from build123d import *

# Parameters (mm, degrees)
ESQUISSE1_R      = 2.5
ESQUISSE1_R_2    = 9
ESQUISSE1_R_3    = 2
EXTRUSION1_DEPTH = 3
CONG_1_R         = 15
EXTRUSION2_REACH = 5
ESQUISSE2_W      = 300
ESQUISSE2_H      = 3
ESQUISSE2_W_2    = 3
ESQUISSE2_H_2    = 91
ESQUISSE2_H_3    = 79
EXTRUSION3_REACH = 5
ESQUISSE3_R      = 2.5


with BuildPart() as part:
    # Esquisse1 → Extrusion1 (new body)
    with BuildSketch(Plane(origin=(0, 0, 0), x_dir=(1, 0, 0), z_dir=(0, 1, 0))):
        Polygon((0, 0), (24, 0), (24, 117), (165, 117), (306, 117), (306, 0), (330, 0), (330, 210), (0, 210), align=None)
        with Locations((10, 200)):
            Circle(ESQUISSE1_R, mode=Mode.SUBTRACT)
        with Locations((320, 200)):
            Circle(ESQUISSE1_R, mode=Mode.SUBTRACT)
        with Locations((10, 99)):
            Circle(ESQUISSE1_R, mode=Mode.SUBTRACT)
        with Locations((320, 99)):
            Circle(ESQUISSE1_R, mode=Mode.SUBTRACT)
        with Locations((10, 10)):
            Circle(ESQUISSE1_R, mode=Mode.SUBTRACT)
        with Locations((320, 10)):
            Circle(ESQUISSE1_R, mode=Mode.SUBTRACT)
        with Locations((40, 170)):
            Circle(ESQUISSE1_R_2, mode=Mode.SUBTRACT)
        with Locations((40, 145)):
            Circle(ESQUISSE1_R_3, mode=Mode.SUBTRACT)
        with Locations((40, 130)):
            Circle(ESQUISSE1_R_3, mode=Mode.SUBTRACT)
    extrude(amount=EXTRUSION1_DEPTH)

    # Congé1
    cong_1_edges = [part.edges().sort_by_distance(p)[0] for p in [
        (0, 1.5, -210),
        (330, 1.5, -210),
        (330, 1.5, 0),
        (0, 1.5, 0),
    ]]
    fillet(cong_1_edges, radius=CONG_1_R)

    # Esquisse2 → Extrusion2 (cut, up to next)
    with BuildSketch(Plane(origin=(0, 3, 0), x_dir=(1, 0, 0), z_dir=(0, 1, 0)), mode=Mode.PRIVATE) as extrusion2_sk1:
        with Locations((165, 208.5)):
            Rectangle(ESQUISSE2_W, ESQUISSE2_H)
    extrusion2_tool1 = extrude(extrusion2_sk1.sketch, amount=-EXTRUSION2_REACH, mode=Mode.PRIVATE) & part.part
    add(extrusion2_tool1.solids().sort_by_distance((165, 3, -208.5))[0], mode=Mode.SUBTRACT)
    # Esquisse2 → Extrusion2 (cut, up to next)
    with BuildSketch(Plane(origin=(0, 3, 0), x_dir=(1, 0, 0), z_dir=(0, 1, 0)), mode=Mode.PRIVATE) as extrusion2_sk2:
        with Locations((1.5, 149.5)):
            Rectangle(ESQUISSE2_W_2, ESQUISSE2_H_2)
    extrusion2_tool2 = extrude(extrusion2_sk2.sketch, amount=-EXTRUSION2_REACH, mode=Mode.PRIVATE) & part.part
    add(extrusion2_tool2.solids().sort_by_distance((1.5, 3, -149.5))[0], mode=Mode.SUBTRACT)
    # Esquisse2 → Extrusion2 (cut, up to next)
    with BuildSketch(Plane(origin=(0, 3, 0), x_dir=(1, 0, 0), z_dir=(0, 1, 0)), mode=Mode.PRIVATE) as extrusion2_sk3:
        with Locations((1.5, 54.5)):
            Rectangle(ESQUISSE2_W_2, ESQUISSE2_H_3)
    extrusion2_tool3 = extrude(extrusion2_sk3.sketch, amount=-EXTRUSION2_REACH, mode=Mode.PRIVATE) & part.part
    add(extrusion2_tool3.solids().sort_by_distance((1.5, 3, -54.5))[0], mode=Mode.SUBTRACT)
    # Esquisse2 → Extrusion2 (cut, up to next)
    with BuildSketch(Plane(origin=(0, 3, 0), x_dir=(1, 0, 0), z_dir=(0, 1, 0)), mode=Mode.PRIVATE) as extrusion2_sk4:
        with Locations((328.5, 54.5)):
            Rectangle(ESQUISSE2_W_2, ESQUISSE2_H_3)
    extrusion2_tool4 = extrude(extrusion2_sk4.sketch, amount=-EXTRUSION2_REACH, mode=Mode.PRIVATE) & part.part
    add(extrusion2_tool4.solids().sort_by_distance((328.5, 3, -54.5))[0], mode=Mode.SUBTRACT)
    # Esquisse2 → Extrusion2 (cut, up to next)
    with BuildSketch(Plane(origin=(0, 3, 0), x_dir=(1, 0, 0), z_dir=(0, 1, 0)), mode=Mode.PRIVATE) as extrusion2_sk5:
        with Locations((328.5, 149.5)):
            Rectangle(ESQUISSE2_W_2, ESQUISSE2_H_2)
    extrusion2_tool5 = extrude(extrusion2_sk5.sketch, amount=-EXTRUSION2_REACH, mode=Mode.PRIVATE) & part.part
    add(extrusion2_tool5.solids().sort_by_distance((328.5, 3, -149.5))[0], mode=Mode.SUBTRACT)

    # Esquisse3 → Extrusion3 (cut, up to next)
    with BuildSketch(Plane(origin=(0, 3, 0), x_dir=(1, 0, 0), z_dir=(0, 1, 0)), mode=Mode.PRIVATE) as extrusion3_sk1:
        with Locations((31, 195)):
            Circle(ESQUISSE3_R)
    extrusion3_tool1 = extrude(extrusion3_sk1.sketch, amount=-EXTRUSION3_REACH, mode=Mode.PRIVATE) & part.part
    add(extrusion3_tool1.solids().sort_by_distance((31, 3, -195))[0], mode=Mode.SUBTRACT)
    # Esquisse3 → Extrusion3 (cut, up to next)
    with BuildSketch(Plane(origin=(0, 3, 0), x_dir=(1, 0, 0), z_dir=(0, 1, 0)), mode=Mode.PRIVATE) as extrusion3_sk2:
        with Locations((15, 179)):
            Circle(ESQUISSE3_R)
    extrusion3_tool2 = extrude(extrusion3_sk2.sketch, amount=-EXTRUSION3_REACH, mode=Mode.PRIVATE) & part.part
    add(extrusion3_tool2.solids().sort_by_distance((15, 3, -179))[0], mode=Mode.SUBTRACT)
    # Esquisse3 → Extrusion3 (cut, up to next)
    with BuildSketch(Plane(origin=(0, 3, 0), x_dir=(1, 0, 0), z_dir=(0, 1, 0)), mode=Mode.PRIVATE) as extrusion3_sk3:
        with Locations((15, 120)):
            Circle(ESQUISSE3_R)
    extrusion3_tool3 = extrude(extrusion3_sk3.sketch, amount=-EXTRUSION3_REACH, mode=Mode.PRIVATE) & part.part
    add(extrusion3_tool3.solids().sort_by_distance((15, 3, -120))[0], mode=Mode.SUBTRACT)
    # Esquisse3 → Extrusion3 (cut, up to next)
    with BuildSketch(Plane(origin=(0, 3, 0), x_dir=(1, 0, 0), z_dir=(0, 1, 0)), mode=Mode.PRIVATE) as extrusion3_sk4:
        with Locations((15, 78)):
            Circle(ESQUISSE3_R)
    extrusion3_tool4 = extrude(extrusion3_sk4.sketch, amount=-EXTRUSION3_REACH, mode=Mode.PRIVATE) & part.part
    add(extrusion3_tool4.solids().sort_by_distance((15, 3, -78))[0], mode=Mode.SUBTRACT)
    # Esquisse3 → Extrusion3 (cut, up to next)
    with BuildSketch(Plane(origin=(0, 3, 0), x_dir=(1, 0, 0), z_dir=(0, 1, 0)), mode=Mode.PRIVATE) as extrusion3_sk5:
        with Locations((15, 31)):
            Circle(ESQUISSE3_R)
    extrusion3_tool5 = extrude(extrusion3_sk5.sketch, amount=-EXTRUSION3_REACH, mode=Mode.PRIVATE) & part.part
    add(extrusion3_tool5.solids().sort_by_distance((15, 3, -31))[0], mode=Mode.SUBTRACT)
    # Esquisse3 → Extrusion3 (cut, up to next)
    with BuildSketch(Plane(origin=(0, 3, 0), x_dir=(1, 0, 0), z_dir=(0, 1, 0)), mode=Mode.PRIVATE) as extrusion3_sk6:
        with Locations((299, 195)):
            Circle(ESQUISSE3_R)
    extrusion3_tool6 = extrude(extrusion3_sk6.sketch, amount=-EXTRUSION3_REACH, mode=Mode.PRIVATE) & part.part
    add(extrusion3_tool6.solids().sort_by_distance((299, 3, -195))[0], mode=Mode.SUBTRACT)
    # Esquisse3 → Extrusion3 (cut, up to next)
    with BuildSketch(Plane(origin=(0, 3, 0), x_dir=(1, 0, 0), z_dir=(0, 1, 0)), mode=Mode.PRIVATE) as extrusion3_sk7:
        with Locations((315, 179)):
            Circle(ESQUISSE3_R)
    extrusion3_tool7 = extrude(extrusion3_sk7.sketch, amount=-EXTRUSION3_REACH, mode=Mode.PRIVATE) & part.part
    add(extrusion3_tool7.solids().sort_by_distance((315, 3, -179))[0], mode=Mode.SUBTRACT)
    # Esquisse3 → Extrusion3 (cut, up to next)
    with BuildSketch(Plane(origin=(0, 3, 0), x_dir=(1, 0, 0), z_dir=(0, 1, 0)), mode=Mode.PRIVATE) as extrusion3_sk8:
        with Locations((315, 120)):
            Circle(ESQUISSE3_R)
    extrusion3_tool8 = extrude(extrusion3_sk8.sketch, amount=-EXTRUSION3_REACH, mode=Mode.PRIVATE) & part.part
    add(extrusion3_tool8.solids().sort_by_distance((315, 3, -120))[0], mode=Mode.SUBTRACT)
    # Esquisse3 → Extrusion3 (cut, up to next)
    with BuildSketch(Plane(origin=(0, 3, 0), x_dir=(1, 0, 0), z_dir=(0, 1, 0)), mode=Mode.PRIVATE) as extrusion3_sk9:
        with Locations((315, 78)):
            Circle(ESQUISSE3_R)
    extrusion3_tool9 = extrude(extrusion3_sk9.sketch, amount=-EXTRUSION3_REACH, mode=Mode.PRIVATE) & part.part
    add(extrusion3_tool9.solids().sort_by_distance((315, 3, -78))[0], mode=Mode.SUBTRACT)
    # Esquisse3 → Extrusion3 (cut, up to next)
    with BuildSketch(Plane(origin=(0, 3, 0), x_dir=(1, 0, 0), z_dir=(0, 1, 0)), mode=Mode.PRIVATE) as extrusion3_sk10:
        with Locations((315, 31)):
            Circle(ESQUISSE3_R)
    extrusion3_tool10 = extrude(extrusion3_sk10.sketch, amount=-EXTRUSION3_REACH, mode=Mode.PRIVATE) & part.part
    add(extrusion3_tool10.solids().sort_by_distance((315, 3, -31))[0], mode=Mode.SUBTRACT)


solid = part.part
Read the model definition and answer for the solid it produces. Units are mm, in the model's axes. Coordinates: 2 decimals unless noted, no trailing zeros. Write each loop counter-clockwise with the first axis right and the second up, starting at its lowest first coordinate (ties: lowest second). Pieces come first, ordered by that corner, then holes. Notation, with made-up numbers: (38.5, 62.5) - (94.5, 62.5) arc R20 ccw to (94.5, 72.5) - close; hole circle Ø11 at (-30.75, 45). An arc over 180 degrees is marked (long way). One line per question, with ' | ' between items.
Q1. Find section B-B, the plane z = -170. Write down the section's boundary in (x, y).
Result set:
outline: (3, 0) - (31, 0) - (31, 3) - (3, 3) - close; (49, 0) - (327, 0) - (327, 3) - (49, 3) - close
Q2. Find section C-C, the plane y = 2.2. State how many separate pieces and enclosed holes the cut face has, plus the area to 3 significant figures.
Result set:
separate pieces: 1 | enclosed holes: 19 | area: 33,600 mm^2
Q3. Determine the mould class of faces 1 (the cylindrical face through (4.51, 1.52, -4.28)), 2 (the cylindrical face through (325.49, 1.52, -205.72)), 3 (the cylindrical face through (38.828, 1.479, -178.923)) for opening direction X: +X half, -X half, draft (parallel to the pull), parting line (faces both ways), or undercut.
Result set:
face 1: -X half | face 2: +X half | face 3: undercut
Q4. Consider L1, parallel to X at y = 2.2, z = -120; L2, parallel to X at y = 1.4, z = -31.5; L3, parallel to X at y = 2.45, z = -119.5. Determine where each line is inside the solid, lowest interval first. Write a range as [from, to].
Result set:
L1: [3, 12.5], [17.5, 312.5], [317.5, 327] | L2: [3, 12.55], [17.45, 24], [306, 312.55], [317.45, 327] | L3: [3, 12.55], [17.45, 312.55], [317.45, 327]
Q5. Find section A-A, the plane z = -40. Write down the section's boundary in (x, y).
Result set:
outline: (3, 0) - (24, 0) - (24, 3) - (3, 3) - close; (306, 0) - (327, 0) - (327, 3) - (306, 3) - close
Q6. Each of these flat-tipped pins is pushed along its axis until it touches: P1, Ø0.9, axis at y = 1, z = -46, coming from the +X side; P2, Ø6, axis at x = 15, z = -179, coming from the -Y side; P3, Ø1, axis at x = 99.5, y = 1, coming from the +Z side; P4, Ø0.9, axis at y = 1, z = -47, coming from the -X side. Where does it stop, or does it pass through?
Result set:
P1: x = 327 | P2: y = 0 | P3: z = -117 | P4: x = 3
